Part model, mm, in its own coordinate system. Round coordinates to 2 decimals unless told otherwise and drop trailing zeros. Write each loop counter-clockwise with the first axis right and the second up, starting at its lowest first coordinate (ties: lowest second). Pieces come first, ordered by that corner, then holes.
1) Saw through at B-B on x = 27.5. Write the cut outline in (y, z).
2) Drill centre lines: L1, parallel to X at y = -0.35, z = -3; L2, parallel to X at y = -0.85, z = -17; L3, parallel to Z at x = 73, y = -0.8. Where is each one in solid material? Low to high.
3) Saw through at D-D on x = 68. Write the cut outline in (y, z).
4) Saw through at A-A on y = -0.4. Count the separate pieces of the cut face and the enclosed holes in it, and give its area (3 significant figures).
Autodesk Inventor part; units mm, degrees
ref_plane "YZ Plane" through (0, 0, 0) normal (1, 0, 0) x (0, 1, 0)
ref_plane "XZ Plane" through (0, 0, 0) normal (0, 1, 0) x (-1, 0, 0)
ref_plane "XY Plane" through (0, 0, 0) normal (0, 0, 1) x (1, 0, 0)
sketch "Sketch1" plane through (0, 0, 0) normal (0, 1, 0) x (-1, 0, 0)
  line L0 (-0.4496, -21) -> (-0.4496, 0)
  line L1 (-52.7289, -21) -> (-52.7289, 0)
  circle A0 centre (-44.5893, -10.5) radius 2
  circle A1 centre (-26.5893, -10.5) radius 2
  circle A2 centre (-8.5893, -10.5) radius 2
  circle A3 centre (12.165, -10.5) radius 1.05
  circle A4 centre (26.215, -10.5) radius 1.05
  circle A5 centre (19.19, -3.475) radius 1.05
  circle A6 centre (19.19, -17.525) radius 1.05
  circle A7 centre (19.19, -10.5) radius 3.85
  circle A8 centre (-72.3686, -10.5) radius 2.75
  circle A9 centre (-72.3686, -17.6) radius 1.05
  circle A10 centre (-79.4686, -10.5) radius 1.05
  circle A11 centre (-72.3686, -3.4) radius 1.05
  circle A12 centre (-65.2686, -10.5) radius 1.05
  arc A13 (19.6402, -20.2396) -> (19.6402, -0.7604) centre (19.19, -10.5) ccw
  line L2 (3.19, -21) -> (19.6402, -20.2396)
  line L3 (19.6402, -0.7604) -> (3.19, 0)
  line L4 (-56.3686, 0) -> (3.19, 0)
  line L5 (3.19, -21) -> (-56.3686, -21)
  line L6 (-72.8188, -0.7604) -> (-56.3686, 0)
  arc A14 (-72.8188, -0.7604) -> (-72.8188, -20.2396) centre (-72.3686, -10.5) ccw
  line L7 (-56.3686, -21) -> (-72.8188, -20.2396)
  line L8 (-53.1786, -21) -> (-53.1786, 0)
  line L9 (-52.2793, 0) -> (-52.2793, -21)
  line L10 (-0.8993, -21) -> (-0.8993, 0)
  line L11 (0, 0) -> (0, -21)
extrude "Plate1" add sketch "Sketch1" against normal blind 1.5
equation "\"d0\" = Thickness"
equation "\"BendReliefWidth\" = Thickness"
equation "\"BendReliefDepth\" = 0.5 * Thickness"
equation "\"CornerReliefSize\" = 4 * Thickness"
equation "\"MinimumRemnant\" = 2 * Thickness"
equation "\"TransitionRadius\" = BendRadius"
equation "\"JacobiRadiusSize\" = BendRadius"
equation "\"GapSize\" = Thickness"
properties part number "CAM_ㄷ_frame_1" material "Aluminum 6061"
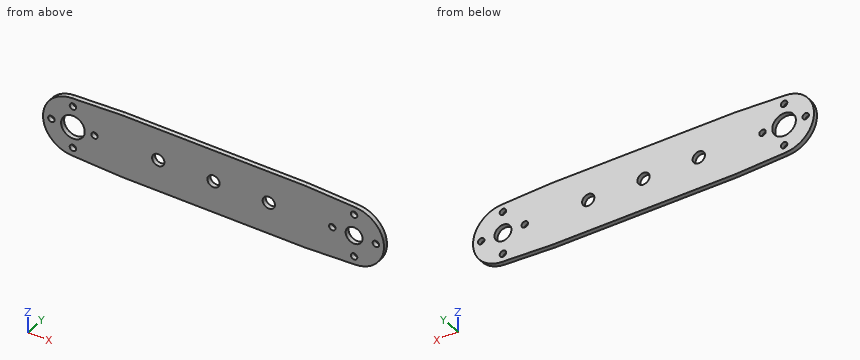
Completed:
1. outline: (-1.5, -21) - (0, -21) - (0, -12.28) - (-1.5, -12.28) - close; (-1.5, -8.72) - (0, -8.72) - (0, 0) - (-1.5, 0) - close
2. L1: x = -25.42 to -20.13, -18.25 to 71.4, 73.34 to 78.6
2. L2: x = -26.46 to -20.1, -18.28 to 71.51, 73.23 to 79.64
2. L3: z = -20.23 to -18.44, -16.76 to -13.18, -7.82 to -4.24, -2.56 to -0.77
3. outline: (-1.5, -20.46) - (0, -20.46) - (0, -0.54) - (-1.5, -0.54) - close
4. separate pieces: 1
4. enclosed holes: 13
4. area: 2,060 mm2
